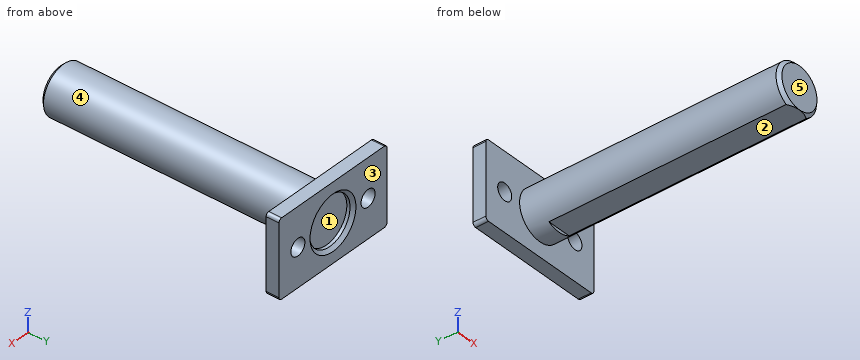
from build123d import *

# Parameters (mm, degrees)
F0_W     = 40
F0_H     = 24
F0_R     = 7.5
F1_DEPTH = 2
F2_DEPTH = 83
F4_D     = 5.2
F4_DEPTH = 15
F4_TIP   = 1.5622376095
F6_DEPTH = 75
F8_DEPTH = 75
F9_SIZE  = 0.99999
F10_R    = 1


# Not quite as in the source:
# - a fillet or chamfer is up to 0.001 mm smaller than in the source, because OpenCascade refuses the exact size


with BuildPart() as f1:
    # F0 (on Front) → F1 (new body, symmetric)
    with BuildSketch(Plane.XZ):
        Rectangle(F0_W, F0_H)
        Circle(F0_R, mode=Mode.SUBTRACT)
    extrude(amount=F1_DEPTH, both=True)

    # F0 (on Front) → F2 (join)
    with BuildSketch(Plane.XZ):
        Circle(F0_R)
    extrude(amount=F2_DEPTH)

    # F4
    with Locations(Plane(origin=(0, 2, 0), x_dir=(-1, 0, 0), z_dir=(0, 1, 0))):
        with Locations((-13, 0), (13, 0)):
            Hole(F4_D / 2, depth=F4_DEPTH)
            with Locations((0, 0, -(F4_DEPTH + F4_TIP / 2))):  # 118° drill point
                Cone(0, F4_D / 2, F4_TIP, mode=Mode.SUBTRACT)

    # F5 (on Front) → F6 (cut)
    with BuildSketch(Plane.XZ):
        with BuildLine():
            Line((3.7416573868, -6.5), (-3.7416573868, -6.5))
            ThreePointArc((-3.7416573868, -6.5), (0, -7.5), (3.7416573868, -6.5))
        make_face()
    extrude(amount=-F6_DEPTH, mode=Mode.SUBTRACT)

    # F7 (on face) → F8 (cut)
    with BuildSketch(Plane.XZ.offset(83)):
        with BuildLine():
            ThreePointArc((-3.7416573868, -6.5), (0, -7.5), (3.7416573868, -6.5))
            Line((3.7416573868, -6.5), (-3.7416573868, -6.5))
        make_face()
    extrude(amount=-F8_DEPTH, mode=Mode.SUBTRACT)

    # F9 (size 1 in the source; OpenCascade refuses exactly that, so slightly less here)
    f9_edges = [f1.edges().sort_by_distance(p)[0] for p in [
        (-7.5, 2, 0),
        (-3.754169, -83, 6.492782),
    ]]
    chamfer(f9_edges, length=F9_SIZE)

    # F10
    f10_edges = [f1.edges().sort_by_distance(p)[0] for p in [
        (20, 0, 12),
        (-20, 0, 12),
        (20, 0, -12),
        (-20, 0, -12),
    ]]
    fillet(f10_edges, radius=F10_R)


solid = f1.part
For this review, take the finished solid that the model builds, in its own axes (mm). Face numbers are marked on the shaded views. A direction names the side the tool comes from. Give positions to 0.01 mm unless a question says otherwise; leave off trailing zeros. Loops run counter-clockwise (first coordinate to the right, second up) from the corner with the lowest first, then second, coordinate; pieces in that order, holes last.
Item 1: Take a section at A-A, the plane x = -13. State the section outline as (y, z) points, and give its area (3 significant figures).
Item 2: Insertion check: pin 1 (3.5 mm diameter, centred on x = -1, y = -48, fed in from -Z); pin 2 (6 mm diameter, centred on x = -8.5, y = -12, fed in from -Z); pin 3 (10 mm diameter, centred on x = 11, y = -33.5, fed in from +Z); pin 4 (3 mm diameter, centred on x = -13, z = 0, fed in from +Y). Each pin has a flat end and moves straight along its axis. Give the tip position at first contact, or say it passes through.
Item 3: For line 1 along Z through (x, y) = (0, 0.35); line 2 along Y through (x, z) = (-10.5, -4); line 3 along X through (y, z) = (-18, 0.25), list the stretches that pass through material, from the lowest coordinate up.
Item 4: Take a section at C-C, the plane z = -1.5. Give the number of separate pieces and of enclosed holes in the cut face, and give its area (3 significant figures).
Item 5: Take a section at B-B, the plane y = -56.5. State the section outline as (x, z) points, and give its area (3 significant figures).
Item 6: Draft analysis for pull direction Z (two halves, no side actions). For the marked faces 1, 2 and 3, state which applies: +Z half, -Z half, draft (parallel to the pull), parting line (faces both ways), or undercut.
Item 7: Tool access review of the marked faces 4 and 5: name each direction out of +Z, -Z, +X, -X, +Y, -Y from which nothing blocks a thin tool from reaching the whole face with its end or side.
Calculated:
1. outline: (-2, -12) - (2, -12) - (2, -2.6) - (-2, -2.6) - close; (-2, 2.6) - (2, 2.6) - (2, 12) - (-2, 12) - close
1. area: 75.2 mm2
2. pin 1: stops at z = -6.5
2. pin 2: stops at z = -5.1
2. pin 3: stops at z = 4.5
2. pin 4: passes through
3. line 1: z = -12 to -7.5, 7.5 to 12
3. line 2: y = -2 to 2
3. line 3: x = -7.5 to 7.5
4. separate pieces: 3
4. enclosed holes: 0
4. area: 1,290 mm2
5. outline: (-3.74, -6.5) - (3.74, -6.5) arc R7.5 ccw (long way) to start
5. area: 172 mm2
6. face 1: undercut
6. face 2: -Z half
6. face 3: draft
7. face 4: -Y
7. face 5: +Z, -Z, +X, -X, -Y
